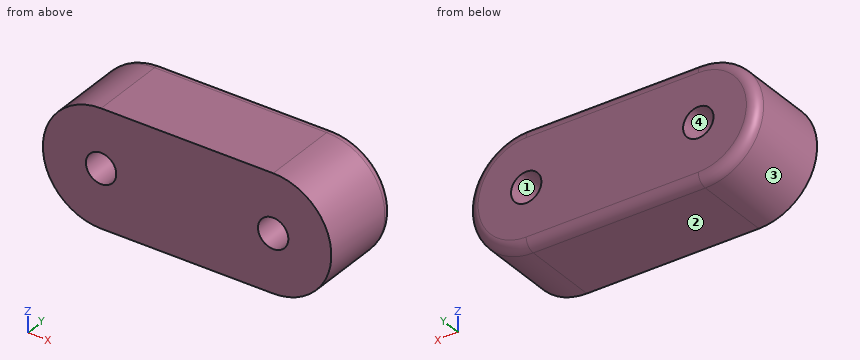
Autodesk Inventor part; units mm, degrees
ref_plane "YZ Plane" through (0, 0, 0) normal (1, 0, 0) x (0, 1, 0)
ref_plane "XZ Plane" through (0, 0, 0) normal (0, 1, 0) x (-1, 0, 0)
ref_plane "XY Plane" through (0, 0, 0) normal (0, 0, 1) x (1, 0, 0)
sketch "Sketch1" plane through (0, 0, 0) normal (0, 1, 0) x (-1, 0, 0)
  line L0 (8.5, 0) -> (-8.5, 0) construction
  line L1 (8.5, 5.75) -> (-8.5, 5.75)
  line L2 (-8.5, -5.75) -> (8.5, -5.75)
  arc A0 (8.5, -5.75) -> (8.5, 5.75) centre (8.5, 0) ccw
  arc A1 (-8.5, 5.75) -> (-8.5, -5.75) centre (-8.5, 0) ccw
  circle A2 centre (-8.5, 0) radius 1.5
  circle A3 centre (8.5, 0) radius 1.5
  point P0 (0, 0)
  dimension "d0" = 11.5
  dimension "d1" = 17
  dimension "d2" = 3
  dimension "d3" = 3
extrude "Extrusion1" add sketch "Sketch1" along normal blind 8.5
thread "Thread1"
thread "Thread2"
fillet "Fillet1" radius 1 4 edges at (0, 8.5, 5.75) (14.25, 8.5, 0) (0, 8.5, -5.75) (-14.25, 8.5, 0)
properties part number "SolderSupportDoubleNut" material "Brass"
Model file for the job. Use its own axes, mm. Face numbers are marked on the shaded views. Coordinates: 2 decimals unless noted, no trailing zeros. Loops run counter-clockwise (first coordinate to the right, second up) from the corner with the lowest first, then second, coordinate; pieces in that order, holes last. Notation, with made-up numbers: M -17,50.5 L 32,50.5 A25 cw 32,72.5 Z; hole C 33.25,2.5 d4. An arc over 180 degrees is marked long. Use CSV: the item, a comma, the result in double quotes. Start each with the question number.
1. Band-saw the part on C-C, the plane y = 6.5. List the corners of the cut face in (x, z).
2. Band-saw the part on B-B, the plane x = 7.75. List the corners of the cut face in (y, z), then the cut area to 3 significant figures.
3. Band-saw the part on A-A, the plane z = 0. List the corners of the cut face in (x, y).
4. Two-plate mould, pull along Z, no slides. Class the marked faces 1, 2, 3 and 4: pulls with the +Z half, pulls with the -Z half, needs draft (parallel to the pull), parting line crosses it, or undercut.
5. Flat gauge pins, fed straight in: pin 1 (3 mm diameter, centred on y = 6.5, z = -3, fed in from -X); pin 2 (1 mm diameter, centred on y = 5.5, z = -4, fed in from +X). Where does each tip first touch, or does it go through?
6. Probe probe 1 along Z at (x, y) = (-8.5, 2.75); probe 2 along X at (y, z) = (1, -1.25). List the from-to ranges inside material, lowest first. Write a range as [from, to].
Entries:
1,outline,"M -8.5,-5.75 L 8.5,-5.75 A5.75 ccw 8.5,5.75 L -8.5,5.75 A5.75 ccw Z; hole C -8.5,0 d3; hole C 8.5,0 d3"
2,outline,"M 0,-5.75 L 7.5,-5.75 A1 ccw 8.5,-4.75 L 8.5,-1.3 L 0,-1.3 Z; M 0,1.3 L 8.5,1.3 L 8.5,4.75 A1 ccw 7.5,5.75 L 0,5.75 Z"
2,area,"75.2 mm2"
3,outline,"M -14.25,0 L -10,0 L -10,8.5 L -13.25,8.5 A1 ccw -14.25,7.5 Z; M -7,0 L 7,0 L 7,8.5 L -7,8.5 Z; M 10,0 L 14.25,0 L 14.25,7.5 A1 ccw 13.25,8.5 L 10,8.5 Z"
4,face 1,"undercut"
4,face 2,"pulls with the -Z half"
4,face 3,"parting line crosses it"
4,face 4,"undercut"
5,pin 1,"stops at x = -14.05"
5,pin 2,"stops at x = 13.06"
6,probe 1,"z = [-5.75, -1.5], [1.5, 5.75]"
6,probe 2,"x = [-14.11, -9.33], [-7.67, 7.67], [9.33, 14.11]"
